Build history of the part. All positions in model axes, mm. Round coordinates to 2 decimals unless told otherwise and drop trailing zeros. Write each loop counter-clockwise with the first axis right and the second up, starting at its lowest first coordinate (ties: lowest second). Pieces come first, ordered by that corner, then holes.
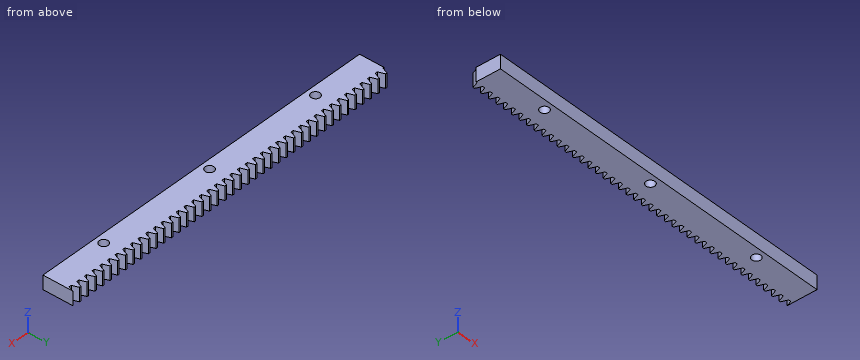
from build123d import *

# Parameters (mm, degrees)
BLANKSKE_W              = 130
BLANKSKE_H              = 11
BLANK_DEPTH             = 5
TOOTHCUTSIM_DEPTH       = 131.560330882
TEETHCUTS_COUNT         = 42
TEETHCUTS_PITCH         = 3.14159265
ESQUISSE1_R             = 1.6
ENL_V_MAT_EXTRU_1_DEPTH = 10


with BuildPart() as part:
    # BlankSke → Blank (new body)
    with BuildSketch(Plane.XY):
        with Locations((65, 5.5)):
            Rectangle(BLANKSKE_W, BLANKSKE_H)
    extrude(amount=-BLANK_DEPTH)

    # TooCutSkeSim → ToothCutSim (cut, through all)
    with BuildSketch(Plane.XY):
        Polygon((0.44443537, 8.75), (-0.44443537, 8.75), (-1.272613241, 11.0254), (1.272613241, 11.0254), align=None)
    toothcutsim = extrude(amount=-TOOTHCUTSIM_DEPTH, mode=Mode.SUBTRACT)

    # TeethCuts: ToothCutSim ×42
    with Locations(*[(i * TEETHCUTS_PITCH, 0, 0) for i in range(1, TEETHCUTS_COUNT)]):
        add(toothcutsim, mode=Mode.SUBTRACT)

    # Esquisse1 → Enlèv. mat.-Extru.1 (cut)
    with BuildSketch(Plane.XY):
        with Locations((21.5, 3)):
            Circle(ESQUISSE1_R)
        with Locations((65, 3)):
            Circle(ESQUISSE1_R)
        with Locations((108.5, 3)):
            Circle(ESQUISSE1_R)
    extrude(amount=-ENL_V_MAT_EXTRU_1_DEPTH, mode=Mode.SUBTRACT)


solid = part.part
1) Slice it at A-A (y = 3). Write the cut outline in (x, z).
Results:
outline: (0, -5) - (19.9, -5) - (19.9, 0) - (0, 0) - close; (23.1, -5) - (63.4, -5) - (63.4, 0) - (23.1, 0) - close; (66.6, -5) - (106.9, -5) - (106.9, 0) - (66.6, 0) - close; (110.1, -5) - (130, -5) - (130, 0) - (110.1, 0) - close
2) Wall check: L1, parallel to X at y = 4.25, z = -0.65; L2, parallel to X at y = 3.5, z = -3.3; L3, parallel to Y at x = 25, z = -2.05. Give the ranges that are in metal, low to high.
Results:
L1: x = 0 to 20.5, 22.5 to 64, 66 to 107.5, 109.5 to 130
L2: x = 0 to 19.98, 23.02 to 63.48, 66.52 to 106.98, 110.02 to 130
L3: y = 0 to 8.75
3) Slice it at B-B (z = -0.95). Count the separate pieces of the cut face and the enclosed holes in it, plus the area to 3 significant figures.
Results:
separate pieces: 1
enclosed holes: 3
area: 1,250 mm2
4) Pin check, flat tips, straight feed: pin 1 Ø4 at (x, y) = (108.5, 3) entering from -Z; pin 2 Ø0.7 at (x, z) = (122.5, -3.5) entering from +Y. Stop position of each tip, or through.
Results:
pin 1: stops at z = -5
pin 2: stops at y = 8.75
